from build123d import *

# Parameters (mm, degrees)
SKETCH1_W           = 25
SKETCH1_H           = 17
BOSS_EXTRUDE1_DEPTH = 3
SKETCH2_R           = 1.5
BOSS_EXTRUDE2_DEPTH = 8
FILLET3_R           = 1


with BuildPart() as part:
    # Sketch1 → Boss-Extrude1 (new body)
    with BuildSketch(Plane(origin=(0, 0, 0), x_dir=(1, 0, 0), z_dir=(0, 1, 0))):
        Rectangle(SKETCH1_W, SKETCH1_H)
    extrude(amount=BOSS_EXTRUDE1_DEPTH)

    # Sketch2 → Boss-Extrude2 (add)
    with BuildSketch(Plane(origin=(0, 3, 0), x_dir=(1, 0, 0), z_dir=(0, 1, 0))):
        with Locations((-10.5, -6.5)):
            Circle(SKETCH2_R)
        with Locations((10.5, -6.5)):
            Circle(SKETCH2_R)
        with Locations((10.5, 5.999999892)):
            Circle(SKETCH2_R)
        with Locations((-10.5, 5.999999892)):
            Circle(SKETCH2_R)
    extrude(amount=BOSS_EXTRUDE2_DEPTH)

    # Fillet3
    fillet3_edges = [part.edges().sort_by_distance(p)[0] for p in [
        (0, 0, 8.5),
        (-12.5, 0, 0),
        (0, 0, -8.5),
        (12.5, 0, 0),
    ]]
    fillet(fillet3_edges, radius=FILLET3_R)


solid = part.part
The model under review builds one solid part; all positions refer to its coordinate system, in mm. A direction names the side the tool comes from. Coordinates: 2 decimals unless noted, no trailing zeros. Loops run counter-clockwise (first coordinate to the right, second up) from the corner with the lowest first, then second, coordinate; pieces in that order, holes last. Notation, with made-up numbers: M 65.25,49.25 L 79.25,49.25 A30 ccw 79.25,78.25 Z; hole C 41.25,-23.75 d6. An arc over 180 degrees is marked long. Put each result on its own line as item: value. Start each with the question number.
Q1. For faces 1 (the cylindrical face through (0.175, 0.301, -8.215)), 2 (the cylindrical face through (-11.7, 6.9, 7.4)), list the 3-axis set-ups (+Z, -Z, +X, -X, +Y, -Y) from which the entire face can be reached by the end or side of a thin tool; tool diameter is ignored.
Q2. The part is to be moulded in two halves that separate along X. For faces 3 (the cylindrical face through (9.3, 6.9, 7.4)), 4 (the flat face through (-11, 11, 6)), 5 (the cylindrical face through (-12.215, 0.301, -0.119)), say which applies: +X half, -X half, draft (parallel to the pull), parting line (faces both ways), or undercut.
Q3. Add section D-D (x = 10.5). Write out the cut boundary in (y, z), and give its area (3 significant figures).
Q4. Add section B-B (x = -5.5). Write out the cut boundary in (y, z), and give its area (3 significant figures).
Q5. Add section A-A (z = -6). Write out the cut boundary in (x, y), and give its area (3 significant figures).
Q6. Wall thickness on line 1 (X direction, y = 10.75, z = 6.5); line 2 (Y direction, x = 3.5, z = -2.25); line 3 (X direction, y = 4.75, z = 7.75): over which ranges is each line inside the solid? List them lowest first.
Q7. Add section C-C (y = 9.75). Write out the cut boundary in (x, z).
Q8. Clearance check with flat-ended pins moving along their axes: pin 1 (5 mm diameter, centred on x = 0.5, z = -3, fed in from +Y); pin 2 (1.5 mm diameter, centred on y = 5, z = -1.5, fed in from -X). State where each tip first meets the part, or that it passes through.
Answers:
1. face 1: -Z, +X, -X, -Y
1. face 2: +Y
2. face 3: undercut
2. face 4: draft
2. face 5: -X half
3. outline: M 0,-7.5 A1 ccw 1,-8.5 L 3,-8.5 L 3,-7.5 L 11,-7.5 L 11,-4.5 L 3,-4.5 L 3,5 L 11,5 L 11,8 L 3,8 L 3,8.5 L 1,8.5 A1 ccw 0,7.5 Z
3. area: 98.6 mm^2
4. outline: M 0,-7.5 A1 ccw 1,-8.5 L 3,-8.5 L 3,8.5 L 1,8.5 A1 ccw 0,7.5 Z
4. area: 50.6 mm^2
5. outline: M -12.5,1 A1 ccw -11.5,0 L 11.5,0 A1 ccw 12.5,1 L 12.5,3 L 12,3 L 12,11 L 9,11 L 9,3 L -9,3 L -9,11 L -12,11 L -12,3 L -12.5,3 Z
5. area: 123 mm^2
6. line 1: x = -12 to -9, 9 to 12
6. line 2: y = 0 to 3
6. line 3: x = -11.33 to -9.67, 9.67 to 11.33
7. outline: C -10.5,-6 d3; C -10.5,6.5 d3; C 10.5,-6 d3; C 10.5,6.5 d3
8. pin 1: stops at y = 3
8. pin 2: passes through
